Check sheet for the modelled part. Datum: model origin and axes. Units: mm. Face numbers are marked on the shaded views. A direction names the side the tool comes from. Coordinates: 2 decimals unless noted, no trailing zeros. Loops run counter-clockwise (first coordinate to the right, second up) from the corner with the lowest first, then second, coordinate; pieces in that order, holes last. Notation, with made-up numbers: M 15,-36 L 29,-36 A19 ccw 29,-30 Z; hole C 71,82 d4. An arc over 180 degrees is marked long. Answer as CSV lines item,"result". Start each with the question number.
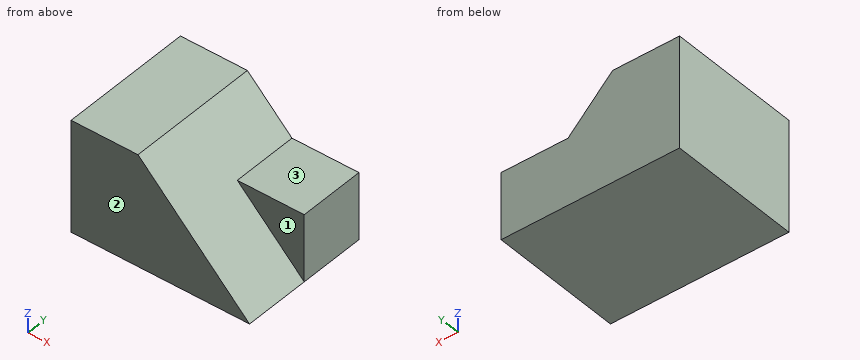
from build123d import *

# Parameters (mm, degrees)
F0_W     = 50.8
F0_H     = 31.75
F1_DEPTH = 38.1
F3_DEPTH = 38.1
F5_DEPTH = 19.05


with BuildPart() as f1:
    # F0 (on Front) → F1 (new body)
    with BuildSketch(Plane.XZ):
        with Locations((25.4, 15.875)):
            Rectangle(F0_W, F0_H)
    extrude(amount=-F1_DEPTH)

    # F2 (on face) → F3 (cut)
    with BuildSketch(Plane.XZ):
        Polygon((19.05, 31.75), (50.8, 0), (50.8, 31.75), align=None)
    extrude(amount=-F3_DEPTH, mode=Mode.SUBTRACT)

    # F4 (on face) → F5 (join)
    with BuildSketch(Plane(origin=(0, 38.1, 0), x_dir=(-1, 0, 0), z_dir=(0, 1, 0))):
        Polygon((-50.8, 19.05), (-50.8, 0), (-31.75, 19.05), align=None)
    extrude(amount=-F5_DEPTH)


solid = f1.part
Item 1: Sectioned sample at A-A, the plane x = 33. Record the boundary of the cut face in (y, z), and give its area (3 significant figures).
Item 2: Material ranges on line 1 (Y direction, x = 47, z = 19); line 2 (Z direction, x = 47.5, y = 31); line 3 (X direction, y = 33, z = 29), recorded low to high. Write a range as from..to.
Item 3: Sectioned sample at C-C, the plane y = 17. Record the boundary of the cut face in (x, z).
Item 4: Set-up check for the marked faces 1, 2 and 3: record each of +Z, -Z, +X, -X, +Y, -Y from which the full face is reachable in a straight line by a thin tool's end or side.
Item 5: Sectioned sample at B-B, the plane z = 5. Record the boundary of the cut face in (x, y).
Item 6: Sectioned sample at D-D, the plane x = 22.5. Record the boundary of the cut face in (y, z), and give its area (3 significant figures).
Item 7: Go/stop test with flat-tipped pins: pin 1 (9.5 mm diameter, centred on x = 43.5, y = 32, fed in from +Z); pin 2 (8 mm diameter, centred on y = 9, z = 27, fed in from +X). Record where each tip stops, or that it passes through.
Reply:
1,outline,"M 0,0 L 38.1,0 L 38.1,19.05 L 19.05,19.05 L 19.05,17.8 L 0,17.8 Z"
1,area,"702 mm²"
2,line 1,"19.05..38.1"
2,line 2,"0..19.05"
2,line 3,"0..21.8"
3,outline,"M 0,0 L 50.8,0 L 19.05,31.75 L 0,31.75 Z"
4,face 1,"+Z, +X, -Y"
4,face 2,"+Z, -Z, +X, -X, -Y"
4,face 3,"+Z, +X, +Y, -Y"
5,outline,"M 0,0 L 45.8,0 L 45.8,19.05 L 50.8,19.05 L 50.8,38.1 L 0,38.1 Z"
6,outline,"M 0,0 L 38.1,0 L 38.1,28.3 L 0,28.3 Z"
6,area,"1,080 mm²"
7,pin 1,"z = 19.05"
7,pin 2,"x = 27.8"
